Design review of the part built by this model. Coordinates are the model's own, in mm. Face numbers are marked on the shaded views. Coordinates: 2 decimals unless noted, no trailing zeros. Loops run counter-clockwise (first coordinate to the right, second up) from the corner with the lowest first, then second, coordinate; pieces in that order, holes last. Notation, with made-up numbers: M 13,-21.5 L 58,-21.5 A24 ccw 58,-4.5 Z; hole C 5,-9 d9. An arc over 180 degrees is marked long. Put each result on its own line as item: value. Start each with the question number.
(1) Take a section at A-A, the plane x = 0. Give the boundary of the cut face in (y, z), then the cut area to 3 significant figures.
(2) Take a section at B-B, the plane z = 2.5. Give the boundary of the cut face in (x, y), then the cut area to 3 significant figures.
(3) The part is to be moulded in two halves that separate along Y. For the marked faces 1, 2 and 3, say which applies: +Y half, -Y half, draft (parallel to the pull), parting line (faces both ways), or undercut.
(4) For probe 1 along Y at (x, z) = (0, 3.55); probe 2 along Z at (x, y) = (3, -7); probe 3 along Y at (x, z) = (-3.5, 3.3), list the stretches that pass through material, from the lowest coordinate up. Write a range as [from, to].
(5) Take a section at D-D, the plane x = -3.5. Give the boundary of the cut face in (y, z), then the cut area to 3 significant figures.
(6) Take a section at C-C, the plane y = 0. Give the boundary of the cut face in (x, z), then the cut area to 3 significant figures.
```python
from build123d import *

# Parameters (mm, degrees)
SKETCH1_W           = 26
SKETCH1_H           = 20
BOSS_EXTRUDE1_DEPTH = 5
SKETCH2_R           = 2.5
CUT_EXTRUDE1_DEPTH  = 5
CUT_EXTRUDE2_REACH  = 30.302
SKETCH3_R           = 1.5


with BuildPart() as part:
    # Sketch1 → Boss-Extrude1 (new body)
    with BuildSketch(Plane.XY):
        Rectangle(SKETCH1_W, SKETCH1_H)
    extrude(amount=BOSS_EXTRUDE1_DEPTH)

    # Sketch2 → Cut-Extrude1 (cut)
    with BuildSketch(Plane.XY.offset(5)):
        Circle(SKETCH2_R)
    extrude(amount=-CUT_EXTRUDE1_DEPTH, mode=Mode.SUBTRACT)

    # Sketch3 → Cut-Extrude2 (cut, up to next)
    with BuildSketch(Plane.ZY.offset(13), mode=Mode.PRIVATE) as cut_extrude2_sk1:
        with Locations((2.5, 7)):
            Circle(SKETCH3_R)
    cut_extrude2_tool1 = extrude(cut_extrude2_sk1.sketch, amount=-CUT_EXTRUDE2_REACH, mode=Mode.PRIVATE) & part.part
    # Sketch3 → Cut-Extrude2 (cut, up to next)
    with BuildSketch(Plane.ZY.offset(13), mode=Mode.PRIVATE) as cut_extrude2_sk2:
        with Locations(Location((2.5, -7, 0), (0, 0, 270))):
            Circle(SKETCH3_R)
    cut_extrude2_tool2 = extrude(cut_extrude2_sk2.sketch, amount=-CUT_EXTRUDE2_REACH, mode=Mode.PRIVATE) & part.part
    add(cut_extrude2_tool1.solids().sort_by_distance((-13, 7, 2.5))[0], mode=Mode.SUBTRACT)
    add(cut_extrude2_tool2.solids().sort_by_distance((-13, -7, 2.5))[0], mode=Mode.SUBTRACT)


solid = part.part
```
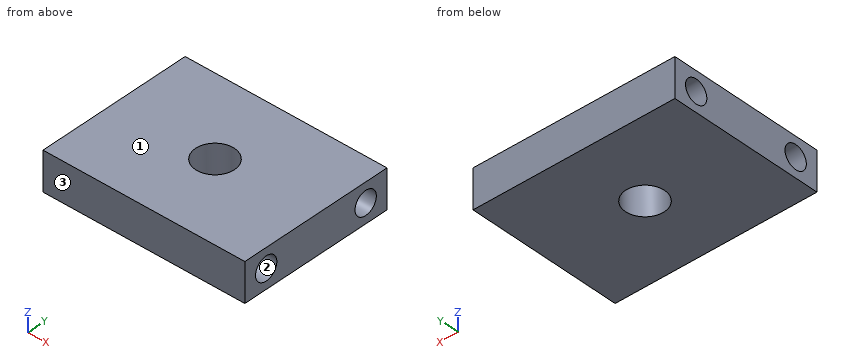
Computed values:
1. outline: M -10,0 L -2.5,0 L -2.5,5 L -10,5 Z; M 2.5,0 L 10,0 L 10,5 L 2.5,5 Z; hole C -7,2.5 d3; hole C 7,2.5 d3
1. area: 60.9 mm^2
2. outline: M -13,-10 L 13,-10 L 13,-8.5 L -13,-8.5 Z; M -13,-5.5 L 13,-5.5 L 13,5.5 L -13,5.5 Z; M -13,8.5 L 13,8.5 L 13,10 L -13,10 Z; hole C 0,0 d5
2. area: 344 mm^2
3. face 1: draft
3. face 2: undercut
3. face 3: -Y half
4. probe 1: y = [-10, -8.07], [-5.93, -2.5], [2.5, 5.93], [8.07, 10]
4. probe 2: z = [0, 1], [4, 5]
4. probe 3: y = [-10, -8.27], [-5.73, 5.73], [8.27, 10]
5. outline: M -10,0 L 10,0 L 10,5 L -10,5 Z; hole C -7,2.5 d3; hole C 7,2.5 d3
5. area: 85.9 mm^2
6. outline: M -13,0 L -2.5,0 L -2.5,5 L -13,5 Z; M 2.5,0 L 13,0 L 13,5 L 2.5,5 Z
6. area: 105 mm^2
